Autodesk Inventor part; units mm, degrees
ref_plane "YZ Plane" through (0, 0, 0) normal (1, 0, 0) x (0, 1, 0)
ref_plane "XZ Plane" through (0, 0, 0) normal (0, 1, 0) x (-1, 0, 0)
ref_plane "XY Plane" through (0, 0, 0) normal (0, 0, 1) x (1, 0, 0)
sketch "Эскиз2" plane through (0, 0, 0) normal (0, 1, 0) x (-1, 0, 0)
  line L0 (0, 0) -> (-58, 0)
  line L1 (-58, 0) -> (-58, 37)
  line L2 (-58, 37) -> (0, 37)
  line L3 (0, 37) -> (0, 0)
  line L4 (-58, 8) -> (-50, 8)
  line L5 (-50, 8) -> (-50, 0)
  line L6 (-50, 0) -> (-58, 0)
  line L7 (-58, 0) -> (-58, 8)
  line L8 (-58, 37) -> (-47, 37)
  line L9 (-47, 37) -> (-47, 27)
  line L10 (-47, 27) -> (-58, 27)
  line L11 (-58, 27) -> (-58, 37)
  line L12 (-50, 27) -> (-58, 27)
  line L13 (-58, 27) -> (-58, 31.5)
  line L14 (-58, 31.5) -> (-50, 31.5)
  line L15 (-50, 31.5) -> (-50, 27)
  line L16 (0, 37) -> (-11, 37)
  line L17 (-11, 37) -> (-11, 27)
  line L18 (-11, 27) -> (0, 27)
  line L19 (0, 27) -> (0, 37)
  line L20 (-11, 27) -> (-7.6324, 27)
  line L21 (-11, 31.5) -> (-11, 27)
  line L22 (0, 27) -> (-8, 27)
  line L23 (-8, 27) -> (-8, 31.5)
  line L24 (-8, 31.5) -> (0, 31.5)
  line L25 (0, 31.5) -> (0, 27)
  line L26 (-8, 8) -> (0, 8)
  line L27 (0, 8) -> (0, 0)
  line L28 (0, 0) -> (-8, 0)
  line L29 (-8, 0) -> (-8, 8)
  point P0 (0, 31.5)
  dimension "d0" = 58
  dimension "d1" = 37
  dimension "d2" = 8
  dimension "d3" = 8
  dimension "d4" = 10
  dimension "d5" = 11
  dimension "d6" = 4.5
  dimension "d7" = 10
  dimension "d8" = 11
  dimension "d9" = 8
extrude "Выдавливание1" add sketch "Эскиз2" along normal blind 2 contours L0 L5 L4 L1 L10 L9 L2 L17 L18 L3 L26 L29 | L18 L23 L24 L3 | L1 L14 L15 L10
sketch "Эскиз3" plane through (0, 2, 0) normal (0, 1, 0) x (1, 0, 0)
  line L0 (0, -31.5) -> (8, -31.5)
  line L1 (0, -8) -> (0, -31.5)
  line L2 (8, -31.5) -> (0, -31.5)
  line L3 (0, -31.5) -> (0, -29.5)
  line L4 (0, -29.5) -> (8, -29.5)
  line L5 (8, -29.5) -> (8, -31.5)
  line L6 (50, -31.5) -> (58, -31.5)
  line L7 (58, -31.5) -> (58, -8)
  line L8 (50, -31.5) -> (58, -31.5)
  line L9 (58, -31.5) -> (58, -29.5)
  line L10 (58, -29.5) -> (50, -29.5)
  line L11 (50, -29.5) -> (50, -31.5)
  line L12 (50, 0) -> (8, 0)
  line L13 (8, 0) -> (8, -8)
  line L14 (50, 0) -> (8, 0)
  line L15 (8, 0) -> (8, -2)
  line L16 (8, -2) -> (50, -2)
  line L17 (50, -2) -> (50, 0)
  point P0 (0, 0)
  dimension "d12" = 2
  dimension "d13" = 2
extrude "Выдавливание2" add sketch "Эскиз3" along normal blind 23
sketch "Эскиз4" plane through (50, 0, 31.5) normal (0, 0, 1) x (1, 0, 0)
  line L0 (-42, 2) -> (-50, 2)
  line L1 (-42, 0) -> (-42, 25)
  line L2 (-42, 2) -> (-42, 25)
  line L3 (0, 0) -> (0, 25)
  circle A0 centre (-45, 18.5) radius 2
  circle A1 centre (-45, 8.5) radius 2
  circle A2 centre (3, 18.5) radius 2
  circle A3 centre (3, 8.5) radius 2
  point P0 (-50, 0)
  point P1 (-42, 13.5)
  point P2 (0, 13.5)
  dimension "d16" = 4
  dimension "d17" = 5
  dimension "d18" = 3
  dimension "d19" = 4
  dimension "d20" = 5
  dimension "d21" = 4
  dimension "d22" = 5
  dimension "d23" = 3
  dimension "d24" = 4
extrude "Выдавливание3" cut sketch "Эскиз4" against normal blind 10
sketch "Эскиз6" plane through (50, 0, 0) normal (0, 0, -1) x (-1, 0, 0)
  line L0 (0, 2) -> (0, 25)
  line L1 (42, 25) -> (0, 25)
  circle A0 centre (24.5, 13.5) radius 1.5
  circle A1 centre (17.5, 13.5) radius 1.5
  circle A2 centre (31.5, 13.5) radius 1.5
  circle A3 centre (38.5, 13.5) radius 1.5
  circle A4 centre (10.5, 13.5) radius 1.5
  circle A5 centre (3.5, 13.5) radius 1.5
  circle A6 centre (10.5, 20.5) radius 1.5
  circle A7 centre (10.5, 6.5) radius 1.5
  circle A8 centre (31.5, 20.5) radius 1.5
  circle A9 centre (31.5, 6.5) radius 1.5
  point P0 (50, 0)
  point P1 (0, 13.5)
  point P2 (21, 25)
  point P3 (21, 13.5)
  dimension "d27" = 3
  dimension "d28" = 3
  dimension "d29" = 3.5
  dimension "d30" = 3.5
  dimension "d31" = 3
  dimension "d32" = 3
  dimension "d33" = 3
  dimension "d34" = 3
  dimension "d35" = 7
  dimension "d36" = 7
  dimension "d37" = 7
  dimension "d38" = 0
  dimension "d39" = 7
  dimension "d40" = 3
  dimension "d41" = 3
  dimension "d42" = 7
  dimension "d43" = 7
  dimension "d44" = 3
  dimension "d45" = 3
extrude "Выдавливание4" cut sketch "Эскиз6" against normal blind 10
sketch "Эскиз7" plane through (0, 2, 0) normal (0, 1, 0) x (1, 0, 0)
  circle A0 centre (5, -13.5) radius 2
  line L0 (8, -2) -> (8, -8)
  line L1 (8, -8) -> (0, -8)
  circle A1 centre (5, -23.5) radius 2
  circle A2 centre (53, -13.5) radius 2
  line L2 (50, -8) -> (50, -2)
  circle A3 centre (53, -23.5) radius 2
  line L3 (8, -2) -> (50, -2)
  circle A4 centre (29, -14) radius 4
  line L4 (11, -37) -> (47, -37)
  circle A5 centre (40, -25) radius 4
  line L5 (58, -29.5) -> (58, -8)
  circle A6 centre (18, -25) radius 4
  line L6 (0, -8) -> (0, -29.5)
  circle A7 centre (25, -25) radius 1.5
  circle A8 centre (33, -25) radius 1.5
  circle A9 centre (40, -32) radius 1.5
  circle A10 centre (47, -25) radius 1.5
  circle A11 centre (11, -25) radius 1.5
  circle A12 centre (18, -18) radius 1.5
  circle A13 centre (40, -18) radius 1.5
  circle A14 centre (18, -32) radius 1.5
  circle A15 centre (29, -21) radius 1.5
  circle A16 centre (36, -14) radius 1.5
  circle A17 centre (22, -14) radius 1.5
  circle A18 centre (29, -7) radius 1.5
  point P0 (0, 0)
  point P1 (29, -2)
  dimension "d48" = 4
  dimension "d49" = 3
  dimension "d50" = 5.5
  dimension "d51" = 4
  dimension "d52" = 10
  dimension "d53" = 4
  dimension "d54" = 3
  dimension "d55" = 4
  dimension "d56" = 8
  dimension "d57" = 23
  dimension "d58" = 8
  dimension "d59" = 12
  dimension "d60" = 18
  dimension "d61" = 8
  dimension "d62" = 18
  dimension "d63" = 3
  dimension "d64" = 3
  dimension "d65" = 3
  dimension "d66" = 3
  dimension "d67" = 3
  dimension "d68" = 3
  dimension "d69" = 7
  dimension "d70" = 7
  dimension "d71" = 7
  dimension "d72" = 7
  dimension "d73" = 7
  dimension "d74" = 7
  dimension "d75" = 3
  dimension "d76" = 3
  dimension "d77" = 3
  dimension "d78" = 3
  dimension "d79" = 3
  dimension "d80" = 3
  dimension "d81" = 7
  dimension "d82" = 7
  dimension "d83" = 7
  dimension "d84" = 7
extrude "Выдавливание5" cut sketch "Эскиз7" against normal blind 10
fillet "Сопряжение1" radius 2 13 edges at (58, 25, 30.5) (50, 25, 30.5) (50, 25, 1) (8, 25, 1) (8, 25, 30.5) (0, 25, 30.5) (54, 0, 31.5) (4, 0, 31.5) (29, 0, 0) (58, 1, 8) (0, 1, 8) (11, 1, 37) (47, 1, 37)
properties material "Сталь"
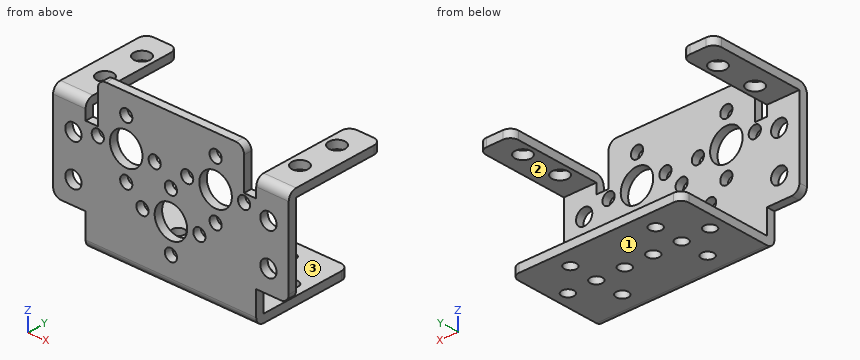
Here's how the part is built. I have some questions about the finished solid (model axes, mm). Face numbers are marked on the shaded views. A direction names the side the tool comes from. Round coordinates to 2 decimals unless told otherwise and drop trailing zeros. Order: outer loops, then holes, each group sorted by start corner. A loop starts at its lowest first (then second) coordinate and runs counter-clockwise, first axis right, second up. Notation, with made-up numbers: M 19,86 L 46,86 A14 ccw 46,94 Z; hole C 3,-39.75 d10. An arc over 180 degrees is marked long. Answer in a Markdown table with one row per item.
Item 1: For the marked faces 1, 2 and 3, which set-ups out of +Z, -Z, +X, -X, +Y, -Y let a thin tool reach every point of the face, with its end or its side?
A:
| item | result |
|---|---|
| face 1 | -Z, +X, -X, +Y, -Y |
| face 2 | -Z, +X, -X, +Y |
| face 3 | +Z, +X, -X, +Y |
Item 2: Imagine slicing it at B-B, the plane y = 13.5. State how many separate pieces and enclosed holes the cut face has, and give its area (3 significant figures).
A:
| item | result |
|---|---|
| separate pieces | 9 |
| enclosed holes | 0 |
| area | 80.0 mm2 |
Item 3: Imagine slicing it at A-A, the plane y = 3. Write out the boundary of the cut face in (x, z), and give its area (3 significant figures).
A:
| item | result |
|---|---|
| outline | M 0,29.5 L 8,29.5 L 8,31.5 L 0,31.5 Z; M 8,0 L 50,0 L 50,2 L 8,2 Z; M 50,29.5 L 58,29.5 L 58,31.5 L 50,31.5 Z |
| area | 116 mm2 |
Item 4: I'm going to push flat-ended pins straight in: pin 1 (4 mm diameter, centred on x = 22, z = 14, fed in from +Y); pin 2 (1 mm diameter, centred on y = 1, z = 30.5, fed in from -X); pin 3 (6 mm diameter, centred on x = 24.5, y = 20, fed in from +Z); pin 4 (4 mm diameter, centred on x = 52, y = 3, fed in from +Z). Where does each tip first touch, or does it pass through?
A:
| item | result |
|---|---|
| pin 1 | stops at y = 2 |
| pin 2 | stops at x = 0 |
| pin 3 | stops at z = 2 |
| pin 4 | stops at z = 31.5 |
Item 5: If I drill on L1, parallel to X at y = 1.5, z = 32; L2, parallel to Z at x = 5, y = 0.65; L3, parallel to Z at x = 40, y = 1.45, over which ranges is the centre line in solid material (lowest first)? Write a range as from..to.
A:
| item | result |
|---|---|
| L1 | x = 11..16.5, 19.5..38.5, 41.5..47 |
| L2 | z = 8..11.5, 15.5..21.5, 25.5..30.98 |
| L3 | z = 0.08..16.5, 19.5..21, 29..30.5, 33.5..37 |
